Autodesk Inventor part; units mm, degrees
ref_plane "YZ Plane" through (0, 0, 0) normal (1, 0, 0) x (0, 1, 0)
ref_plane "XZ Plane" through (0, 0, 0) normal (0, 1, 0) x (-1, 0, 0)
ref_plane "XY Plane" through (0, 0, 0) normal (0, 0, 1) x (1, 0, 0)
sketch "Sketch1" plane through (0, 0, 0) normal (0, 1, 0) x (-1, 0, 0)
  circle A0 centre (0, 0) radius 38.1
  circle A1 centre (0, 0) radius 3.175
  dimension "d0" = 76.2
  dimension "d1" = 6.35
extrude "Extrusion1" add sketch "Sketch1" along normal blind 12.7
sketch "Sketch2" plane through (0, 12.7, 0) normal (0, 1, 0) x (1, 0, 0)
  circle A0 centre (0, 0) radius 6.35
  circle A1 centre (0, 0) radius 31.75
  dimension "d4" = 63.5
  dimension "d5" = 12.7
extrude "Extrusion2" cut sketch "Sketch2" against normal blind 10.16
properties part number "largeinertiawheel" material "Aluminum 6061"
Build history of the part. All positions in model axes, mm. A direction names the side the tool comes from. Coordinates: 2 decimals unless noted, no trailing zeros. Order: outer loops, then holes, each group sorted by start corner. A loop starts at its lowest first (then second) coordinate and runs counter-clockwise, first axis right, second up.
Item 1: Saw through at A-A on z = 0. List the corners of the cut face in (x, y) (3 decimals), then the cut area to 3 significant figures.
Filled in:
outline: (-38.1, 0) - (-3.175, 0) - (-3.175, 12.7) - (-6.35, 12.7) - (-6.35, 2.54) - (-31.75, 2.54) - (-31.75, 12.7) - (-38.1, 12.7) - close; (3.175, 0) - (38.1, 0) - (38.1, 12.7) - (31.75, 12.7) - (31.75, 2.54) - (6.35, 2.54) - (6.35, 12.7) - (3.175, 12.7) - close
area: 371 mm2
Item 2: Mould opens along X. For faces 1 (the cylindrical face through (-1.38, 7.69, 6.2)), 2 (the cylindrical face through (30.235, 6.261, 23.183)), 3 (the flat face through (-8, 0, 1)) say: released by +X, released by -X, zero draft, split by the parting line, or undercut.
Filled in:
face 1: undercut
face 2: split by the parting line
face 3: zero draft
Item 3: Drill centre lines: L1, parallel to Z at x = 0, y = 6 (3 decimals); L2, parallel to Y at x = 21.5, z = -23; L3, parallel to X at y = 6, z = -16.5. Where is each one in solid material? Low to high.
Filled in:
L1: z = -38.1 to -31.75, -6.35 to -3.175, 3.175 to 6.35, 31.75 to 38.1
L2: y = 0 to 2.54
L3: x = -34.34 to -27.13, 27.13 to 34.34
Item 4: Saw through at C-C on y = 1.5. List the corners of the cut face in (x, z) (3 decimals).
Filled in:
outline: circle Ø76.2 at (0, 0); hole circle Ø6.35 at (0, 0)
Item 5: Saw through at D-D on y = 5.75. List the corners of the cut face in (x, z) (3 decimals).
Filled in:
outline: circle Ø76.2 at (0, 0); circle Ø12.7 at (0, 0); hole circle Ø63.5 at (0, 0); hole circle Ø6.35 at (0, 0)
Item 6: Saw through at B-B on x = 0. List the corners of the cut face in (y, z) (3 decimals).
Filled in:
outline: (0, -38.1) - (12.7, -38.1) - (12.7, -31.75) - (2.54, -31.75) - (2.54, -6.35) - (12.7, -6.35) - (12.7, -3.175) - (0, -3.175) - close; (0, 3.175) - (12.7, 3.175) - (12.7, 6.35) - (2.54, 6.35) - (2.54, 31.75) - (12.7, 31.75) - (12.7, 38.1) - (0, 38.1) - close
Item 7: Drop flat-ended pins along their axis: pin 1 Ø5 at (y, z) = (9.5, 23) entering from -X; pin 2 Ø1.5 at (y, z) = (6, -19) entering from +X; pin 3 Ø1.5 at (y, z) = (5, 19.5) entering from -X; pin 4 Ø5 at (x, z) = (0, 0) entering from -Y. Give the stop position or say it passes through.
Filled in:
pin 1: stops at x = -32.11
pin 2: stops at x = 33.44
pin 3: stops at x = -33.17
pin 4: passes through
Item 8: Tool access for faces 4 (the cylindrical face through (0.69, 6.26, 3.1)), 5 (the cylindrical face through (-6.883, 7.691, 30.995)): list every direction of +Z, -Z, +X, -X, +Y, -Y with a clear straight run to the whole face (end or side of a thin tool).
Filled in:
face 4: +Y, -Y
face 5: +Y
